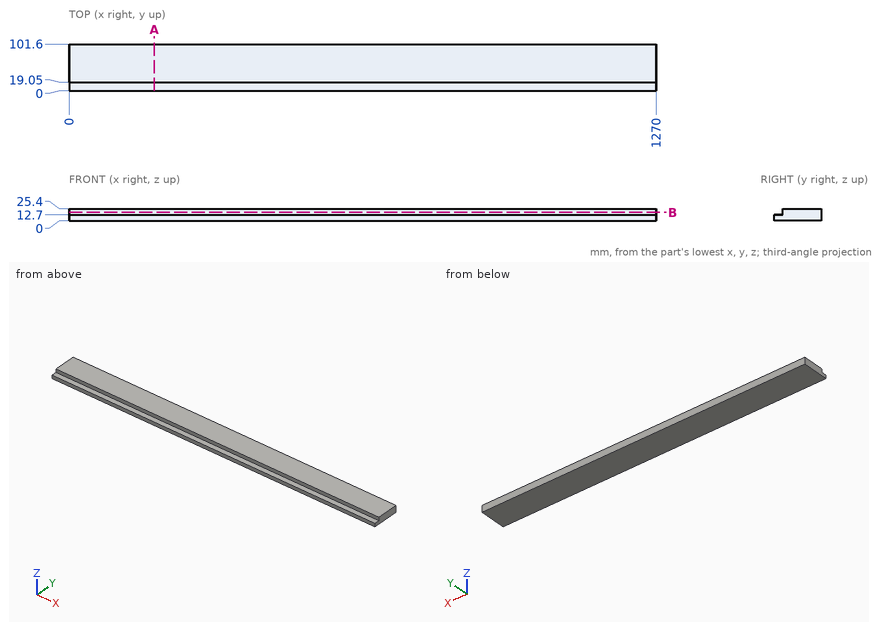
Job drawing, mm, ordinate dimensions from the low corner. One solid piece. Give positions to 0.01 mm unless a question says otherwise; leave off trailing zeros. Loops run counter-clockwise (first coordinate to the right, second up) from the corner with the lowest first, then second, coordinate; pieces in that order, holes last.
Item 1: Flat gauge pins, fed straight in: pin 1 (4 mm diameter, centred on x = 514, z = 21, fed in from -Y); pin 2 (9.5 mm diameter, centred on x = 885.5, y = 7.5, fed in from +Z). Where does each tip first touch, or does it go through?
Answers follow:
pin 1: stops at y = 19.05
pin 2: stops at z = 12.7
Item 2: Slice it at A-A, the plane x = 184.5. List the corners of the cut face in (y, z), and give its area (3 significant figures).
Answers follow:
outline: (0, 0) - (101.6, 0) - (101.6, 25.4) - (19.05, 25.4) - (19.05, 12.7) - (0, 12.7) - close
area: 2,340 mm2
Item 3: Drill centre lines: line 1 (Y direction, x = 854, z = 18.75); line 2 (Z direction, x = 441, y = 4.5). Where is each one in solid material? Low to high.
Answers follow:
line 1: y = 19.05 to 101.6
line 2: z = 0 to 12.7
Item 4: Slice it at B-B, the plane z = 17.75. List the corners of the cut face in (x, y), and give its area (3 significant figures).
Answers follow:
outline: (0, 19.05) - (1270, 19.05) - (1270, 101.6) - (0, 101.6) - close
area: 105,000 mm2
